For this review, take the finished solid that the model builds, in its own axes (mm). A direction names the side the tool comes from. Round coordinates to 2 decimals unless told otherwise and drop trailing zeros. Loops run counter-clockwise (first coordinate to the right, second up) from the corner with the lowest first, then second, coordinate; pieces in that order, holes last.
1) Tool access review of faces 5 (the flat face through (15.24, -10.84, -4.68)), 6 (the cylindrical face through (3.67, -13.05, -2.5)): name each direction out of +Z, -Z, +X, -X, +Y, -Y from which nothing blocks a thin tool from reaching the whole face with its end or side.
2) Insertion check: pin 1 (6 mm diameter, centred on y = -17.5, z = -0.5, fed in from +X); pin 2 (6 mm diameter, centred on x = 7, z = -1.5, fed in from +Y); pin 3 (4 mm diameter, centred on y = 4, z = 2.5, fed in from +X); pin 4 (10 mm diameter, centred on x = -5.5, z = -9.5, fed in from +Y). Each pin has a flat end and moves straight along its axis. Give the tip position at first contact, or say it passes through.
3) Wall thickness on L1, parallel to Z at x = 22.5, y = -3; L2, parallel to Z at x = -2.5, y = -8; L3, parallel to X at y = -7.5, z = 2: over which ranges is each line inside the solid? List them lowest first.
4) Mouldability with a two-part tool opening along Y and no side actions: class faces 1 (the flat face through (8, -5, -13.725)), 2 (the cylindrical face through (2.11, -15.53, 2.99)), 3 (the cylindrical face through (12.914, -5.757, -4.678)), 4 (the flat face through (16.35, -9.03, -4.68)) as pulls with the +Y half, pulls with the -Y half, needs draft (parallel to the pull), parting line crosses it, or undercut.
5) Take a section at C-C (x = 9.5). Give the number of separate pieces and of enclosed holes in the cut face, then the cut area to 3 significant figures.
6) Take a section at A-A (z = -0.25). State the section outline as (x, y) points.
7) Take a section at D-D (z = -7). State the section outline as (x, y) points, then the cut area to 3 significant figures.
8) Take a section at B-B (z = 2). State the section outline as (x, y) points.
```python
from build123d import *

# Parameters (mm, degrees)
SKETCH1_R           = 1.75
BOSS_EXTRUDE1_DEPTH = 15.478309227
SKETCH2_R           = 1.75
BOSS_EXTRUDE2_DEPTH = 10
SKETCH5_W           = 2.4
SKETCH5_H           = 27.5
CUT_EXTRUDE1_DEPTH  = 15.478309227
CUT_EXTRUDE2_DEPTH  = 18.35
FILLET1_R           = 10
CHAMFER1_SIZE       = 0.2


with BuildPart() as part:
    # Sketch1 → Boss-Extrude1 (new body)
    with BuildSketch(Plane(origin=(-2.115260895, 1.332543188, 0), x_dir=(0, 0, -1), z_dir=(0.8461043578704047, -0.533017275135347, 0))):
        with BuildLine():
            Line((16.124998711, 13.75), (1.124998711, 13.75))
            ThreePointArc((1.124998711, 13.75), (-2.94086528, 12.065863992), (-4.625001289, 8))
            Line((-4.625001289, 8), (-4.625001289, -8))
            ThreePointArc((-4.625001289, -8), (-2.94086528, -12.065863992), (1.124998711, -13.75))
            Line((1.124998711, -13.75), (16.124998711, -13.75))
            Line((16.124998711, -13.75), (16.124998711, 13.75))
        make_face()
        with Locations(Location((1.124998711, 8, 0), (0, 0, 90))):
            Circle(SKETCH1_R, mode=Mode.SUBTRACT)
        with Locations(Location((1.124998711, -8, 0), (0, 0, 90))):
            Circle(SKETCH1_R, mode=Mode.SUBTRACT)
    extrude(amount=BOSS_EXTRUDE1_DEPTH)

    # Sketch2 → Boss-Extrude2 (add)
    with BuildSketch(Plane(origin=(10.981003995, -6.91766302, 0), x_dir=(0, 0, -1), z_dir=(0.8461043578704048, -0.5330172751353467, 0))):
        with BuildLine():
            ThreePointArc((-4.625001289, -8), (-2.94086528, -12.065863992), (1.124998711, -13.75))
            Line((1.124998711, -13.75), (13.724998711, -13.75))
            Line((13.724998711, -13.75), (13.724998711, -2.9))
            Line((13.724998711, -2.9), (13.724998711, 0))
            Line((13.724998711, 0), (13.724998711, 2.9))
            Line((13.724998711, 2.9), (13.724998711, 13.75))
            Line((13.724998711, 13.75), (1.124998711, 13.75))
            ThreePointArc((1.124998711, 13.75), (-2.94086528, 12.065863992), (-4.625001289, 8))
            Line((-4.625001289, 8), (-4.625001289, -8))
        make_face()
        with Locations((1.124998711, -8)):
            Circle(SKETCH2_R, mode=Mode.SUBTRACT)
        with Locations((1.124998711, 8)):
            Circle(SKETCH2_R, mode=Mode.SUBTRACT)
    extrude(amount=BOSS_EXTRUDE2_DEPTH)

    # Sketch5 → Cut-Extrude1 (cut)
    with BuildSketch(Plane(origin=(10.981003995, -6.91766302, 0), x_dir=(0, 0, -1), z_dir=(0.8461043578704048, -0.5330172751353467, 0))):
        with Locations((14.924998711, 0)):
            Rectangle(SKETCH5_W, SKETCH5_H)
    extrude(amount=-CUT_EXTRUDE1_DEPTH, mode=Mode.SUBTRACT)

    # Sketch7 → Cut-Extrude2 (cut)
    with BuildSketch(Plane(origin=(0, 0, -13.724998711), x_dir=(-1, 0, 0), z_dir=(0, 0, -1))):
        with BuildLine():
            Line((-16.021823666, -7.58604821), (-16.685981664, -10.511606986))
            Line((-16.685981664, -10.511606986), (-13.760422887, -11.175764984))
            ThreePointArc((-13.760422887, -11.175764984), (-15.634577963, -9.849258033), (-16.021823666, -7.58604821))
        make_face()
        with BuildLine():
            ThreePointArc((-16.021823666, -7.58604821), (-15.634577963, -9.849258033), (-13.760422887, -11.175764984))
            Line((-13.760422887, -11.175764984), (-13.649729888, -10.688171855))
            ThreePointArc((-13.649729888, -10.688171855), (-15.211525784, -9.582749396), (-15.534230536, -7.69674121))
            Line((-15.534230536, -7.69674121), (-16.021823666, -7.58604821))
        make_face()
        with BuildLine():
            ThreePointArc((-15.534230536, -7.69674121), (-15.211525784, -9.582749396), (-13.649729888, -10.688171855))
            Line((-13.649729888, -10.688171855), (-13.605452688, -10.493134603))
            ThreePointArc((-13.605452688, -10.493134603), (-15.042304913, -9.476145941), (-15.339193285, -7.741018409))
            Line((-15.339193285, -7.741018409), (-15.534230536, -7.69674121))
        make_face()
        with BuildLine():
            ThreePointArc((-15.339193285, -7.741018409), (-15.042304913, -9.476145941), (-13.605452688, -10.493134603))
            Line((-13.605452688, -10.493134603), (-13.096264889, -8.250206208))
            Line((-13.096264889, -8.250206208), (-15.339193285, -7.741018409))
        make_face()
        with BuildLine():
            Line((-13.096264889, -8.250206208), (-13.605452688, -10.493134603))
            ThreePointArc((-13.605452688, -10.493134603), (-12.708361538, -10.517259579), (-11.870325157, -10.196246231))
            Line((-11.870325157, -10.196246231), (-13.096264889, -8.250206208))
        make_face()
        with BuildLine():
            ThreePointArc((-14.322204622, -6.304166185), (-14.973602792, -6.921446486), (-15.339193285, -7.741018409))
            Line((-15.339193285, -7.741018409), (-13.096264889, -8.250206208))
            Line((-13.096264889, -8.250206208), (-14.322204622, -6.304166185))
        make_face()
        with BuildLine():
            Line((-10.829211518, -7.862302856), (-13.096264889, -8.250206208))
            Line((-13.096264889, -8.250206208), (-11.870325157, -10.196246231))
            ThreePointArc((-11.870325157, -10.196246231), (-11.082603872, -9.361587919), (-10.796264889, -8.250206208))
            ThreePointArc((-10.796264889, -8.250206208), (-10.804516348, -8.055556207), (-10.829211518, -7.862302856))
        make_face()
        with BuildLine():
            Line((-11.870325157, -10.196246231), (-11.763721702, -10.365467103))
            ThreePointArc((-11.763721702, -10.365467103), (-10.907502914, -9.458229807), (-10.596264889, -8.250206208))
            ThreePointArc((-10.596264889, -8.250206208), (-10.605233866, -8.038630121), (-10.632076442, -7.82857213))
            Line((-10.632076442, -7.82857213), (-10.829211518, -7.862302856))
            ThreePointArc((-10.829211518, -7.862302856), (-10.804516348, -8.055556207), (-10.796264889, -8.250206208))
            ThreePointArc((-10.796264889, -8.250206208), (-11.082603872, -9.361587919), (-11.870325157, -10.196246231))
        make_face()
        with BuildLine():
            Line((-14.322204622, -6.304166185), (-13.096264889, -8.250206208))
            Line((-13.096264889, -8.250206208), (-11.767505167, -6.372868305))
            ThreePointArc((-11.767505167, -6.372868305), (-13.034434615, -5.951037441), (-14.322204622, -6.304166185))
        make_face()
        with BuildLine():
            ThreePointArc((-11.651960844, -6.209621531), (-13.029058069, -5.751109722), (-14.428808077, -6.134945313))
            Line((-14.428808077, -6.134945313), (-14.322204622, -6.304166185))
            ThreePointArc((-14.322204622, -6.304166185), (-13.034434615, -5.951037441), (-11.767505167, -6.372868305))
            Line((-11.767505167, -6.372868305), (-11.651960844, -6.209621531))
        make_face()
        with BuildLine():
            Line((-11.767505167, -6.372868305), (-13.096264889, -8.250206208))
            Line((-13.096264889, -8.250206208), (-10.829211518, -7.862302856))
            ThreePointArc((-10.829211518, -7.862302856), (-11.150224866, -7.024266475), (-11.767505167, -6.372868305))
        make_face()
    extrude(amount=-CUT_EXTRUDE2_DEPTH, mode=Mode.SUBTRACT)

    # Fillet1
    fillet1_edges = [part.edges().sort_by_distance(p)[0] for p in [
        (1.334405806, -17.091581212, -13.724998711),
        (15.992380872, 6.176288629, -13.724998711),
    ]]
    fillet(fillet1_edges, radius=FILLET1_R)

    # Chamfer1
    # the kernel refuses this chamfer: 0.2 mm, written as the material it adds along each edge
    with BuildSketch(Plane(origin=(14.428808077, -6.134945313, -13.724998711), x_dir=(-0.533017275135546, -0.8461043578702794, 0), z_dir=(0, 0, 1))) as chamfer1_piece_1_section:
        with BuildLine():
            Line((CHAMFER1_SIZE, 0), (0.007427842, -0.192572158))
            ThreePointArc((0.007427842, -0.192572158), (0.001963813, -0.09907174), (0, 0))
            Line((0, 0), (CHAMFER1_SIZE, 0))
        make_face()
    chamfer1_piece_1 = extrude(amount=18.35, mode=Mode.PRIVATE)
    chamfer1_piece_1 = chamfer1_piece_1 - Plane(origin=(13.096264889, -8.250206208, -13.724998711), x_dir=(0.5330172751353905, 0.8461043578703773, 0), z_dir=(0, 0, -1)) * Cylinder(2.3, 38, mode=Mode.PRIVATE)
    add(chamfer1_piece_1)
    with BuildSketch(Plane(origin=(11.763721702, -10.365467103, -13.724998711), x_dir=(-0.8249315284266814, 0.5652326719215895, 0), z_dir=(0, 0, 1))) as chamfer1_piece_2_section:
        with BuildLine():
            Line((0.192715357, 0), (CHAMFER1_SIZE * 0.0385430714682, -CHAMFER1_SIZE * 0.999256939752))
            Line((CHAMFER1_SIZE * 0.0385430714682, -CHAMFER1_SIZE * 0.999256939752), (0, 0))
            ThreePointArc((0, 0), (0.099073815, 0.001856175), (0.192715357, 0))
        make_face()
    chamfer1_piece_2 = extrude(amount=18.35, mode=Mode.PRIVATE)
    chamfer1_piece_2 = chamfer1_piece_2 - Plane(origin=(13.096264889, -8.250206208, -13.724998711), x_dir=(0.22138599930385242, -0.9751862587794369, 0), z_dir=(0, 0, -1)) * Cylinder(2.3, 38, mode=Mode.PRIVATE)
    add(chamfer1_piece_2)


solid = part.part
```
Response:
1. face 5: +Z, -Z
1. face 6: none
2. pin 1: stops at x = 18.02
2. pin 2: stops at y = 12.97
2. pin 3: stops at x = 21.01
2. pin 4: stops at y = 3.9
3. L1: z = -11.94 to -2.1, -0.15 to 4.44
3. L2: z = -12.73 to -2.87, 0.62 to 4.62
3. L3: x = -7.68 to 10.92, 15.27 to 22.43
4. face 1: needs draft
4. face 2: pulls with the -Y half
4. face 3: undercut
4. face 4: undercut
5. separate pieces: 1
5. enclosed holes: 2
5. area: 506 mm2
6. outline: (-9.41, -10.24) - (12.15, -23.83) - (14.37, -20.3) - (-7.19, -6.72) - close; (-5.57, -4.15) - (15.99, -17.73) - (22.9, -6.76) - (1.34, 6.82) - close; (2.96, 9.38) - (24.51, -4.2) - (26.74, -0.67) - (5.18, 12.91) - close; hole (10.63, -7.83) arc R2.5 ccw to (11.6, -10.26) - (11.87, -10.2) arc R2.3 ccw to (13.61, -10.49) - (13.76, -11.18) - (16.69, -10.51) - (16.02, -7.59) - (15.34, -7.74) arc R2.3 ccw to (14.32, -6.3) - (14.26, -6.04) arc R2.5 ccw to (11.65, -6.21) - (11.77, -6.37) arc R2.3 ccw to (10.83, -7.86) - close
7. outline: (-9.15, -9.83) - (12.41, -23.42) - (26.48, -1.08) - (4.92, 12.5) - close; hole (10.63, -7.83) arc R2.5 ccw to (11.6, -10.26) - (11.87, -10.2) arc R2.3 ccw to (13.61, -10.49) - (13.76, -11.18) - (16.69, -10.51) - (16.02, -7.59) - (15.34, -7.74) arc R2.3 ccw to (14.32, -6.3) - (14.26, -6.04) arc R2.5 ccw to (11.65, -6.21) - (11.77, -6.37) arc R2.3 ccw to (10.83, -7.86) - close
7. area: 650 mm2
8. outline: (-8.95, -9.52) - (12.61, -23.1) - (26.28, -1.4) - (4.72, 12.19) - close; hole (10.63, -7.83) arc R2.5 ccw to (11.6, -10.26) - (11.87, -10.2) arc R2.3 ccw to (13.61, -10.49) - (13.76, -11.18) - (16.69, -10.51) - (16.02, -7.59) - (15.34, -7.74) arc R2.3 ccw to (14.32, -6.3) - (14.26, -6.04) arc R2.5 ccw to (11.65, -6.21) - (11.77, -6.37) arc R2.3 ccw to (10.83, -7.86) - close
